For this review, take the finished solid that the model builds, in its own axes (mm). Round coordinates to 2 decimals unless told otherwise and drop trailing zeros. Write each loop counter-clockwise with the first axis right and the second up, starting at its lowest first coordinate (ties: lowest second). Pieces come first, ordered by that corner, then holes. Notation, with made-up numbers: (79, 10.5) -> (88, 10.5) arc R20 cw to (88, 17.5) -> close; hole circle Ø3 at (24, 24). An arc over 180 degrees is marked (long way). Write item = value, one per line. Start each with the question number.
```python
from build123d import *

# Parameters (mm, degrees)
SKETCH1_R           = 4.191
BOSS_EXTRUDE1_DEPTH = 3.175
CAVITY1_START       = 3.689049998
CAVITY1_DEPTH       = 9.603434939
FILLET3_R           = 1.27


# Read off the part's stored shape, not the designer's step: Cavity1
with BuildPart() as part:
    # Sketch1 → Boss-Extrude1 (new body)
    with BuildSketch(Plane.XY):
        with BuildLine():
            ThreePointArc((9.406966983, 1.494856913), (0, 9.525), (-9.406966983, 1.494856913))
            Line((-9.406966983, 1.494856913), (-15.24, -35.211766))
            Line((-15.24, -35.211766), (15.24, -35.211766))
            Line((15.24, -35.211766), (9.406966983, 1.494856913))
        make_face()
        Circle(SKETCH1_R, mode=Mode.SUBTRACT)
    extrude(amount=BOSS_EXTRUDE1_DEPTH)

    # Cavity1 outline → Cavity1 (cut)
    with BuildSketch(Plane(origin=(0, 0, 0), x_dir=(0.9955947349362284, 0.032256539947670526, 0.08803771576924041), z_dir=(0.09376099278090663, -0.3425138790307331, -0.9348225066311033)).offset(CAVITY1_START)):
        with BuildLine():
            Line((-14.012226084, 36), (-14.169183947, 34.154693399))
            ThreePointArc((-14.169183947, 34.154693399), (-1.135248211, 19.965054491), (11.898687525, 34.154693399))
            Line((11.898687525, 34.154693399), (11.741729662, 36))
            Line((11.741729662, 36), (-14.012226084, 36))
        make_face()
    extrude(amount=CAVITY1_DEPTH, mode=Mode.SUBTRACT)

    # Fillet3
    fillet3_edges = [part.edges().sort_by_distance(p)[0] for p in [
        (-15.24, -35.211766, 1.5875),
        (15.24, -35.211766, 1.5875),
    ]]
    fillet(fillet3_edges, radius=FILLET3_R)


solid = part.part
```
1. Draft analysis for pull direction X (two halves, no side actions). For faces 1 (the cylindrical face through (-0.57, -21.2, 0.17)), 2 (the cylindrical face through (14.73, -34.75, 1.61)), 3 (the cylindrical face through (3.997, 1.259, 1.565)), 4 (the flat face through (0, -13, 3.175)), state which applies: +X half, -X half, draft (parallel to the pull), parting line (faces both ways), or undercut.
2. Consider section C-C, the plane y = 6. Give the boundary of the cut face in (x, z) (3 decimals).
3. Consider section B-B, the plane y = -17.5. Give the boundary of the cut face in (x, z) (3 decimals).
4. Wall thickness on L1, parallel to X at y = 1, z = 0.85; L2, parallel to Y at x = 0, z = 0.6 (3 decimals); L3, parallel to X at y = -0.5, z = 3.05: over which ranges is each line inside the solid? List them lowest first. Write a range as from..to.
5. Consider section A-A, the plane y = 0. Give the boundary of the cut face in (x, z) (3 decimals), then the cut area to 3 significant figures.
6. Clearance check with a flat-ended pin moving along its axis: pin 1 Ø6.5 at (x, y) = (0, 0) entering from -Z. State where the tip first meets the part, or that it passes through.
Outcome:
q1.face_1 = undercut
q1.face_2 = +X half
q1.face_3 = undercut
q1.face_4 = draft
q2.outline = (-7.398, 0) -> (7.398, 0) -> (7.398, 3.175) -> (-7.398, 3.175) -> close
q3.outline = (-12.425, 0) -> (12.425, 0) -> (12.425, 3.175) -> (-12.425, 3.175) -> close
q4.L1 = -9.49..-4.07, 4.07..9.49
q4.L2 = -21.054..-4.191, 4.191..9.525
q4.L3 = -9.72..-4.16, 4.16..9.72
q5.outline = (-9.645, 0) -> (-4.191, 0) -> (-4.191, 3.175) -> (-9.645, 3.175) -> close; (4.191, 0) -> (9.645, 0) -> (9.645, 3.175) -> (4.191, 3.175) -> close
q5.area = 34.6 mm2
q6.pin_1 = through
